CAD build for the part. Positions are in the model's coordinates, mm. A direction names the side the tool comes from. Coordinates: 2 decimals unless noted, no trailing zeros. Write item = value, one per line. Start each with the question number.
(1) Tool access for faces 4 (the face through (-1.297, 0.939, 31.303)), 5 (the face through (-24.94, 4.16, -24.01)): list every direction of +Z, -Z, +X, -X, +Y, -Y with a clear straight run to the whole face (end or side of a thin tool).
(2) Pull direction Z, two halves, no side cores. Call faces 1 (the face through (-24.01, 4.16, 24.94)), 2 (the face through (-30.235, 3.131, 23.183)), 3 (the face through (-1, 0, -1)): +Z half, -Z half, draft (parallel to the pull), parting line (faces both ways), or undercut.
(3) Band-saw the part on A-A (z = 0). Count the separate pieces of the cut face and the enclosed holes in it, and give its area (3 significant figures).
(4) Flat gauge pins, fed straight in: P1, Ø4, axis at x = -24.5, z = 24, coming from the -Y side; P2, Ø1, axis at y = 5, z = 8, coming from the -X side; P3, Ø3.5, axis at x = -23.57, z = 23.57, coming from the -Y side (3 decimals); P4, Ø1, axis at y = 5, z = 17, coming from the +X side. Where does each tip first touch, or does it go through?
(5) Drill centre lines: line 1 (X direction, y = 0.75, z = 22); line 2 (Z direction, x = 14, y = 5); line 3 (Z direction, x = -24.5, y = 4.5). Where is each one in solid material? Low to high. Write a range as from..to.
```python
from build123d import *

# Parameters (mm, degrees)
SKETCH1_R                                      = 38.1
BOSS_EXTRUDE1_DEPTH                            = 6.35
CBORE_FOR_4_BUTTON_HEAD_CAP_SCREW1_D           = 2.8702
CBORE_FOR_4_BUTTON_HEAD_CAP_SCREW1_CBORE_D     = 4.826
CBORE_FOR_4_BUTTON_HEAD_CAP_SCREW1_CBORE_DEPTH = 1.905
CIRPATTERN1_COUNT                              = 8
SKETCH6_R                                      = 0.396875
CUT_EXTRUDE1_DEPTH                             = 7.35
SKETCH7_R                                      = 0.396875
CIRPATTERN2_COUNT                              = 6


with BuildPart() as part:
    # Sketch1 → Boss-Extrude1 (new body)
    with BuildSketch(Plane(origin=(0, 0, 0), x_dir=(1, 0, 0), z_dir=(0, 1, 0))):
        Circle(SKETCH1_R)
    extrude(amount=BOSS_EXTRUDE1_DEPTH)

    # CBORE for #4 Button Head Cap Screw1 (through all)
    with Locations(Plane(origin=(0, 0, 0), x_dir=(-1, 0, 0), z_dir=(0, -1, 0))):
        with Locations((0, -33.3375)):
            cbore_for_4_button_head_cap_screw1 = CounterBoreHole(CBORE_FOR_4_BUTTON_HEAD_CAP_SCREW1_D / 2, CBORE_FOR_4_BUTTON_HEAD_CAP_SCREW1_CBORE_D / 2, CBORE_FOR_4_BUTTON_HEAD_CAP_SCREW1_CBORE_DEPTH)

    # CirPattern1: CBORE for #4 Button Head Cap Screw1 ×8 about axis
    cirpattern1_axis = Axis((0, 0, 0), (0, 1, 0))
    for i in range(1, CIRPATTERN1_COUNT):
        add(cbore_for_4_button_head_cap_screw1.rotate(cirpattern1_axis, i * 360 / CIRPATTERN1_COUNT), mode=Mode.SUBTRACT)

    # Sketch6 → Cut-Extrude1 (cut, through all)
    with BuildSketch(Plane(origin=(0, 6.35, 0), x_dir=(1, 0, 0), z_dir=(0, 1, 0))):
        with Locations((0, 9.525)):
            Circle(SKETCH6_R)
        with Locations((0, 12.827)):
            Circle(SKETCH6_R)
        with Locations((0, 16.129)):
            Circle(SKETCH6_R)
        with Locations((8.248891971, 4.7625)):
            Circle(SKETCH6_R)
        with Locations((11.108507854, 6.4135)):
            Circle(SKETCH6_R)
        with Locations((13.968123738, 8.0645)):
            Circle(SKETCH6_R)
        with Locations((8.248891971, -4.7625)):
            Circle(SKETCH6_R)
        with Locations((11.108507854, -6.4135)):
            Circle(SKETCH6_R)
        with Locations((13.968123738, -8.0645)):
            Circle(SKETCH6_R)
        with Locations((0, -9.525)):
            Circle(SKETCH6_R)
        with Locations((0, -12.827)):
            Circle(SKETCH6_R)
        with Locations((0, -16.129)):
            Circle(SKETCH6_R)
        with Locations((-8.248891971, -4.7625)):
            Circle(SKETCH6_R)
        with Locations((-11.108507854, -6.4135)):
            Circle(SKETCH6_R)
        with Locations((-13.968123738, -8.0645)):
            Circle(SKETCH6_R)
        with Locations((-8.248891971, 4.7625)):
            Circle(SKETCH6_R)
        with Locations((-11.108507854, 6.4135)):
            Circle(SKETCH6_R)
        with Locations((-13.968123738, 8.0645)):
            Circle(SKETCH6_R)
    extrude(amount=-CUT_EXTRUDE1_DEPTH, mode=Mode.SUBTRACT)

    # Cut-Sweep1: sweep along a curve in space
    with BuildLine() as cut_sweep1_path:
        Line((0, 6.35, -3.175), (0, 0, -4.7625))
    # Sketch7 → Cut-Sweep1 (sweep, cut)
    with BuildSketch(Plane(origin=(0, 6.35, 0), x_dir=(1, 0, 0), z_dir=(0, 1, 0))):
        with Locations((0, 3.175)):
            Circle(SKETCH7_R)
    cut_sweep1 = sweep(path=cut_sweep1_path.line, mode=Mode.SUBTRACT)

    # CirPattern2: Cut-Sweep1 ×6 about axis
    cirpattern2_axis = Axis((0, 6.35, 0), (0, 1, 0))
    for i in range(1, CIRPATTERN2_COUNT):
        add(cut_sweep1.rotate(cirpattern2_axis, i * 360 / CIRPATTERN2_COUNT), mode=Mode.SUBTRACT)


solid = part.part
```
Findings below:
q1.face_4 = -Y
q1.face_5 = +Y, -Y
q2.face_1 = undercut
q2.face_2 = parting line
q2.face_3 = draft
q3.separate_pieces = 3
q3.enclosed_holes = 0
q3.area = 440 mm²
q4.P1 = 0
q4.P2 = -37.35
q4.P3 = 1.905
q4.P4 = 34.34
q5.line_1 = -31.11..-25.4, -21.74..21.74, 25.4..31.11
q5.line_2 = -35.43..-8.46, -7.67..7.67, 8.46..35.43
q5.line_3 = -29.18..-24.67, -22.48..22.48, 24.67..29.18
